from build123d import *

# Parameters (mm, degrees)
PAD018_DEPTH         = 60
POCKET023_DEPTH      = 2.101
SKETCH071_W          = 9.65
SKETCH071_H          = 4.8
PAD020_DEPTH         = 46
SKETCH073_R          = 1.75
POCKET026_DEPTH      = 46.001
SKETCH069_R          = 1.75
POCKET024_DEPTH      = 5.001
SKETCH070_R          = 3
POCKET025_DEPTH      = 2.951
POCKET042_DEPTH      = 49.401
SKETCH072_W          = 5.65
SKETCH072_H          = 2.75
POCKET027_DEPTH      = 35.151
POCKET027_DEPTH_BACK = 35.151
PAD019_DEPTH         = 2
PAD024_DEPTH         = 4


with BuildPart() as part:
    # Sketch066 → Pad018 (new body)
    with BuildSketch(Plane.YZ.offset(-21.698)):
        with BuildLine():
            ThreePointArc((-33.15, 1), (-32.857107, 0.292893), (-32.15, 0))
            Line((-32.15, 0), (32.15, 0))
            ThreePointArc((32.15, 0), (32.857107, 0.292893), (33.15, 1))
            Line((33.15, 46), (33.15, 1))
            Line((33.15, 46), (35.15, 46))
            Line((35.15, 46), (35.15, -2))
            Line((35.15, -2), (32.15, -5))
            Line((32.15, -5), (-32.15, -5))
            Line((-32.15, -5), (-35.15, -2))
            Line((-35.15, -2), (-35.15, 46))
            Line((-35.15, 46), (-33.15, 46))
            Line((-33.15, 46), (-33.15, 1))
        make_face()
    extrude(amount=PAD018_DEPTH)

    # Sketch067 → Pocket023 (cut, through all)
    with BuildSketch(Plane.YZ.offset(-19.598)):
        with BuildLine():
            Line((-34.25, 46), (-34.25, 1))
            ThreePointArc((-34.25, 1), (-33.634924, -0.484924), (-32.15, -1.1))
            Line((-32.15, -1.1), (32.15, -1.1))
            ThreePointArc((32.15, -1.1), (33.634924, -0.484924), (34.25, 1))
            Line((34.25, 1), (34.25, 46))
            Line((34.25, 46), (33.15, 46))
            Line((33.15, 46), (33.15, 1))
            ThreePointArc((32.15, 0), (32.857107, 0.292893), (33.15, 1))
            Line((-32.15, 0), (32.15, 0))
            ThreePointArc((-33.15, 1), (-32.857107, 0.292893), (-32.15, 0))
            Line((-33.15, 46), (-33.15, 1))
            Line((-34.25, 46), (-33.15, 46))
        make_face()
    extrude(amount=-POCKET023_DEPTH, mode=Mode.SUBTRACT)

    # Sketch071 → Pad020 (join)
    with BuildSketch(Plane.XY):
        with Locations((0, 30.75)):
            Rectangle(SKETCH071_W, SKETCH071_H)
        with Locations((0, -30.75)):
            Rectangle(SKETCH071_W, SKETCH071_H)
    extrude(amount=PAD020_DEPTH)

    # Sketch073 → Pocket026 (cut, through all)
    with BuildSketch(Plane.XY):
        with Locations((0, 31.75)):
            Circle(SKETCH073_R)
        with Locations((0, -31.75)):
            Circle(SKETCH073_R)
    extrude(amount=POCKET026_DEPTH, mode=Mode.SUBTRACT)

    # Sketch069 → Pocket024 (cut, through all)
    with BuildSketch(Plane.XY):
        with Locations((-15.348, 15.621)):
            Circle(SKETCH069_R)
        with Locations((31.952, 15.621)):
            Circle(SKETCH069_R)
        with Locations((19.652, 0)):
            Circle(SKETCH069_R)
        with Locations((31.952, -19.431)):
            Circle(SKETCH069_R)
        with Locations((-15.348, -19.431)):
            Circle(SKETCH069_R)
        with BuildLine():
            ThreePointArc((7.625, 25.35), (9.825, 18.009341), (12.025, 25.35))
            Line((12.025, 28.35), (12.025, 25.35))
            ThreePointArc((12.025, 28.35), (9.825, 30.549987), (7.625, 28.35))
            Line((7.625, 28.35), (7.625, 25.35))
        make_face()
        with BuildLine():
            ThreePointArc((12.025, -25.35), (9.825, -18.009341), (7.625, -25.35))
            Line((7.625, -25.35), (7.625, -28.35))
            ThreePointArc((7.625, -28.35), (9.825, -30.549988), (12.025, -28.35))
            Line((12.025, -25.35), (12.025, -28.35))
        make_face()
    extrude(amount=-POCKET024_DEPTH, mode=Mode.SUBTRACT)

    # Sketch070 → Pocket025 (cut, through all)
    with BuildSketch(Plane.XY.offset(-2.05)):
        with Locations((-15.348, 15.621)):
            Circle(SKETCH070_R)
        with Locations((19.652, 0)):
            Circle(SKETCH070_R)
        with Locations((31.952, 15.621)):
            Circle(SKETCH070_R)
        with Locations((-15.348, -19.431)):
            Circle(SKETCH070_R)
        with Locations((31.952, -19.431)):
            Circle(SKETCH070_R)
    extrude(amount=-POCKET025_DEPTH, mode=Mode.SUBTRACT)

    # Sketch → Pocket042 (cut, through all)
    with BuildSketch(Plane.XY.offset(-3.4)):
        with BuildLine():
            ThreePointArc((13.825, 28.35), (9.825, 32.350018), (5.825, 28.35))
            Line((5.825, 28.35), (5.825, 22.009341))
            Line((5.825, 22.009341), (13.825, 22.009341))
            Line((13.825, 22.009341), (13.825, 28.35))
        make_face()
        with BuildLine():
            ThreePointArc((5.825, -28.349974), (9.824987, -32.349956), (13.825, -28.35))
            Line((13.825, -22.009341), (13.825, -28.35))
            Line((5.825, -22.009341), (13.825, -22.009341))
            Line((5.825, -28.349974), (5.825, -22.009341))
        make_face()
    extrude(amount=POCKET042_DEPTH, mode=Mode.SUBTRACT)

    # Sketch072 → Pocket027 (cut, two sides)
    with BuildSketch(Plane.XZ) as pocket027_sk:
        with Locations((0, 40.625)):
            Rectangle(SKETCH072_W, SKETCH072_H)
    extrude(amount=-POCKET027_DEPTH, mode=Mode.SUBTRACT)
    extrude(pocket027_sk.sketch, amount=POCKET027_DEPTH_BACK, mode=Mode.SUBTRACT)

    # Sketch074 → Pad019 (join)
    with BuildSketch(Plane.YZ.offset(38.302)):
        with BuildLine():
            Line((-34.05, 46), (-34.05, 1))
            ThreePointArc((-34.05, 1), (-33.493503, -0.343503), (-32.15, -0.9))
            Line((-32.15, -0.9), (32.15, -0.9))
            ThreePointArc((32.15, -0.9), (33.493503, -0.343503), (34.05, 1))
            Line((34.05, 1), (34.05, 46))
            Line((33.15, 46), (34.05, 46))
            Line((33.15, 1), (33.15, 46))
            ThreePointArc((32.15, 0), (32.857107, 0.292893), (33.15, 1))
            Line((-32.15, 0), (32.15, 0))
            ThreePointArc((-33.15, 1), (-32.857107, 0.292893), (-32.15, 0))
            Line((-33.15, 46), (-33.15, 1))
            Line((-34.05, 46), (-33.15, 46))
        make_face()
    extrude(amount=PAD019_DEPTH)

    # Sketch082 → Pad024 (join)
    with BuildSketch(Plane.YZ.offset(40.302)):
        Polygon((-33.15, 46), (-28.35, 46), (-28.35, 36), (-33.15, 31.2), align=None)
        Polygon((33.15, 46), (28.35, 46), (28.35, 36), (33.15, 31.2), align=None)
    extrude(amount=-PAD024_DEPTH)


solid = part.part
For this review, take the finished solid that the model builds, in its own axes (mm). A direction names the side the tool comes from. Coordinates: 2 decimals unless noted, no trailing zeros. Loops run counter-clockwise (first coordinate to the right, second up) from the corner with the lowest first, then second, coordinate; pieces in that order, holes last. Notation, with made-up numbers: (47.5, -36.75) - (55.5, -36.75) arc R17 cw to (55.5, -10.75) - close; hole circle Ø7 at (36, 4.25). An arc over 180 degrees is marked (long way). Return JSON: item names as keys, results as strings.
Item 1: Mouldability with a two-part tool opening along Y and no side actions: class faces 1 (the flat face through (39, 0, -0.9)), 2 (the flat face through (22, 0, -2.05)), 3 (the flat face through (8, -35.15, 22)) as pulls with the +Y half, pulls with the -Y half, needs draft (parallel to the pull), parting line crosses it, or undercut.
Determined:
{"face 1": "needs draft", "face 2": "undercut", "face 3": "pulls with the -Y half"}
Item 2: Take a section at A-A (z = 15). Give the boundary of the cut face in (x, y) (3 decimals), then the cut area to 3 significant figures.
Determined:
{"outline": "(-21.698, -35.15) - (38.302, -35.15) - (38.302, -34.05) - (40.302, -34.05) - (40.302, -33.15) - (4.825, -33.15) - (4.825, -28.35) - (-4.825, -28.35) - (-4.825, -33.15) - (-19.598, -33.15) - (-19.598, -34.25) - (-21.698, -34.25) - close; (-21.698, 34.25) - (-19.598, 34.25) - (-19.598, 33.15) - (-4.825, 33.15) - (-4.825, 28.35) - (4.825, 28.35) - (4.825, 33.15) - (40.302, 33.15) - (40.302, 34.05) - (38.302, 34.05) - (38.302, 35.15) - (-21.698, 35.15) - close; hole circle Ø3.5 at (0, -31.75); hole circle Ø3.5 at (0, 31.75)", "area": "312 mm2"}
Item 3: For faces 4 (the cylindrical face through (-13.96, 12.96, -3.5)), 5 (the cylindrical face through (9.87, 30.55, -4.19)), 6 (the flat face through (4.825, 31, 23)), 7 (the flat face through (-2, -32, 42)), list the 3-axis set-ups (+Z, -Z, +X, -X, +Y, -Y) from which the entire face can be reached by the end or side of a thin tool; tool diameter is ignored.
Determined:
{"face 4": "-Z", "face 5": "+Z, -Z", "face 6": "+Z", "face 7": "+Y, -Y"}
Item 4: Insertion check: pin 1 (5 mm diameter, centred on x = 9.5, y = 10, fed in from +Z); pin 2 (0.5 mm diameter, centred on y = 26, z = -4, fed in from +X). Each pin has a flat end and moves straight along its axis. Give the tip position at first contact, or say it passes through.
Determined:
{"pin 1": "stops at z = 0", "pin 2": "stops at x = 38.3"}
Item 5: Take a section at C-C (y = 9). Give the boundary of the cut face in (x, z), then the cut area to 3 significant figures.
Determined:
{"outline": "(-21.7, -5) - (38.3, -5) - (38.3, -0.9) - (40.3, -0.9) - (40.3, 0) - (-19.6, 0) - (-19.6, -1.1) - (-21.7, -1.1) - close", "area": "299 mm2"}
Item 6: Take a section at B-B (x = 0). State how many separate pieces and enclosed holes the cut face has, then the cut area to 3 significant figures.
Determined:
{"separate pieces": "5", "enclosed holes": "0", "area": "628 mm2"}
Item 7: For line 1 (Y direction, x = 18, z = 4.5); line 2 (X direction, y = -29.5, z = 35.5) (3 decimals); line 3 (Z direction, x = -4.5, y = 2), list the stretches that pass through material, from the lowest coordinate up.
Determined:
{"line 1": "y = -35.15 to -33.15, 33.15 to 35.15", "line 2": "x = -4.825 to 4.825, 36.302 to 40.302", "line 3": "z = -5 to 0"}
